from build123d import *

# Parameters (mm, degrees)
SKETCH1_R           = 8.255
SKETCH1_W           = 42.529452224
SKETCH1_H           = 12.7
BOSS_EXTRUDE1_DEPTH = 12.7
SKETCH2_R           = 6.35
BOSS_EXTRUDE2_DEPTH = 25.4


with BuildPart() as part:
    # Sketch1 → Boss-Extrude1 (new body)
    with BuildSketch(Plane.XY):
        with BuildLine():
            Line((89.999184934, 12.7), (97.04, 12.7))
            Line((97.04, 12.7), (97.04, -12.7))
            Line((97.04, -12.7), (89.999184934, -12.7))
            ThreePointArc((89.999184934, -12.7), (80.474184934, -3.175), (70.949184934, -12.7))
            Line((70.949184934, -12.7), (0, -12.7))
            Line((0, -12.7), (0, 12.7))
            Line((0, 12.7), (70.949184934, 12.7))
            ThreePointArc((70.949184934, 12.7), (80.474184934, 3.175), (89.999184934, 12.7))
        make_face()
        with Locations((57.297, 0)):
            Circle(SKETCH1_R, mode=Mode.SUBTRACT)
        with Locations((23.301842553, 0)):
            Rectangle(SKETCH1_W, SKETCH1_H, mode=Mode.SUBTRACT)
    extrude(amount=BOSS_EXTRUDE1_DEPTH)

    # Sketch2 → Boss-Extrude2 (add, through all)
    with BuildSketch(Plane(origin=(0, 12.7, 0), x_dir=(1, 0, 0), z_dir=(0, 1, 0))):
        with Locations((0, -6.35)):
            Circle(SKETCH2_R)
    extrude(amount=-BOSS_EXTRUDE2_DEPTH)


solid = part.part
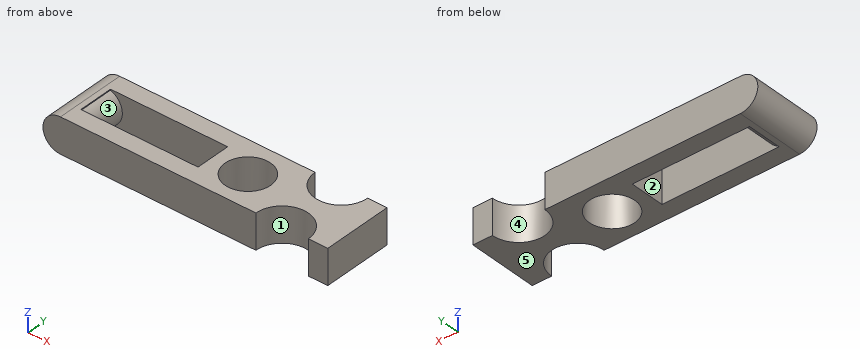
Build history of the part. All positions in model axes, mm. Face numbers are marked on the shaded views. A direction names the side the tool comes from. Coordinates: 2 decimals unless noted, no trailing zeros. Order: outer loops, then holes, each group sorted by start corner. A loop starts at its lowest first (then second) coordinate and runs counter-clockwise, first axis right, second up. Notation, with made-up numbers: (77, -15) - (101, -15) arc R20 cw to (101, 3) - close; hole circle Ø8 at (-16, 27.25). An arc over 180 degrees is marked (long way). Write item = value, one per line. Start each with the question number.
1) Two-plate mould, pull along Y, no slides. Class the marked faces 3, 4 and 5: pulls with the +Y half, pulls with the -Y half, needs draft (parallel to the pull), parting line crosses it, or undercut.
2) Saw through at B-B on y = 0. Write the cut outline in (x, z), then the cut area to 3 significant figures.
3) Saw through at C-C on z = 6.35. Write the cut outline in (x, y) (3 decimals).
4) Flat gauge pins, fed straight in: pin 1 Ø3 at (y, z) = (-9, 9.5) entering from -X; pin 2 Ø4 at (x, y) = (21.5, -2.5) entering from -Z. Where does each tip first touch, or does it go through?
5) Saw through at A-A on x = 9.5. Write the cut outline in (y, z), then the cut area to 3 significant figures.
6) 3-axis set-ups, long thin cutter, end or side, ignore diameter. For the marked faces 1 and 2: which of +Z, -Z, +X, -X, +Y, -Y reach the whole face in a straight line?
7) Wall check: line 1 along Y through (x, z) = (44, 8); line 2 along X through (y, z) = (-6.75, 11.75). Give the ranges that are in metal, low to high. Write a range as from..to.
8) Saw through at D-D on y = 4.75. Write the cut outline in (x, z).
From the geometry:
q1.face_3 = undercut
q1.face_4 = pulls with the +Y half
q1.face_5 = needs draft
q2.outline = (0, 0) - (2.04, 0) - (2.04, 0.34) arc R6.35 ccw to (2.04, 12.36) - (2.04, 12.7) - (0, 12.7) arc R6.35 ccw to start; (44.57, 0) - (49.04, 0) - (49.04, 12.7) - (44.57, 12.7) - close; (65.55, 0) - (97.04, 0) - (97.04, 12.7) - (65.55, 12.7) - close
q2.area = 584 mm^2
q3.outline = (-6.35, -12.7) - (70.949, -12.7) arc R9.525 cw to (89.999, -12.7) - (97.04, -12.7) - (97.04, 12.7) - (89.999, 12.7) arc R9.525 cw to (70.949, 12.7) - (-6.35, 12.7) - close; hole (6.35, -6.35) - (44.567, -6.35) - (44.567, 6.35) - (6.35, 6.35) - close; hole circle Ø16.51 at (57.297, 0)
q4.pin_1 = -6.13
q4.pin_2 = through
q5.outline = (-12.7, 0) - (-6.35, 0) - (-6.35, 12.7) - (-12.7, 12.7) - close; (6.35, 0) - (12.7, 0) - (12.7, 12.7) - (6.35, 12.7) - close
q5.area = 161 mm^2
q6.face_1 = +Z, -Z, -Y
q6.face_2 = +Z, -Z
q7.line_1 = -12.7..-6.35, 6.35..12.7
q7.line_2 = -3.34..52.54, 62.05..73.04, 87.91..97.04
q8.outline = (0, 0) - (2.04, 0) - (2.04, 0.34) arc R6.35 ccw to (2.04, 12.36) - (2.04, 12.7) - (0, 12.7) arc R6.35 ccw to start; (44.57, 0) - (50.55, 0) - (50.55, 12.7) - (44.57, 12.7) - close; (64.05, 0) - (75.23, 0) - (75.23, 12.7) - (64.05, 12.7) - close; (85.72, 0) - (97.04, 0) - (97.04, 12.7) - (85.72, 12.7) - close
